Model file for the job. Use its own axes, mm. Coordinates: 2 decimals unless noted, no trailing zeros. Loops run counter-clockwise (first coordinate to the right, second up) from the corner with the lowest first, then second, coordinate; pieces in that order, holes last. Notation, with made-up numbers: (13, -24) -> (51, -24) arc R33 ccw to (51, 4) -> close; hole circle Ø3 at (30.5, 41). An arc over 180 degrees is marked (long way). Use one line per item in the form item = value.
```python
from build123d import *

# Parameters (mm, degrees)
BOSS_EXTRUDE1_DEPTH     = 25.4
F_1_4_CLEARANCE_HOLE1_D = 6.7564


with BuildPart() as part:
    # Sketch1 → Boss-Extrude1 (new body)
    with BuildSketch(Plane(origin=(0, 0, 0), x_dir=(1, 0, 0), z_dir=(0, 1, 0))):
        with BuildLine():
            Line((-63.5, -66.675), (63.5, -66.675))
            ThreePointArc((63.5, -66.675), (67.990128061, -64.815128061), (69.85, -60.325))
            Line((69.85, -60.325), (69.85, 60.325))
            ThreePointArc((69.85, 60.325), (67.990128061, 64.815128061), (63.5, 66.675))
            Line((63.5, 66.675), (-63.5, 66.675))
            ThreePointArc((-63.5, 66.675), (-67.990128061, 64.815128061), (-69.85, 60.325))
            Line((-69.85, 60.325), (-69.85, -60.325))
            ThreePointArc((-69.85, -60.325), (-67.990128061, -64.815128061), (-63.5, -66.675))
        make_face()
        with BuildLine():
            Line((-55.5625, 41.275), (-33.3375, 41.275))
            ThreePointArc((-33.3375, 41.275), (-32.214967985, 41.739967985), (-31.75, 42.8625))
            Line((-31.75, 42.8625), (-31.75, 52.3875))
            ThreePointArc((-31.75, 52.3875), (-32.214967985, 53.510032015), (-33.3375, 53.975))
            Line((-33.3375, 53.975), (-55.5625, 53.975))
            ThreePointArc((-55.5625, 53.975), (-56.685032015, 53.510032015), (-57.15, 52.3875))
            Line((-57.15, 52.3875), (-57.15, 42.8625))
            ThreePointArc((-57.15, 42.8625), (-56.685032015, 41.739967985), (-55.5625, 41.275))
        make_face(mode=Mode.SUBTRACT)
        with BuildLine():
            Line((-12.7, 42.8625), (-12.7, 52.3875))
            ThreePointArc((-12.7, 52.3875), (-12.235032015, 53.510032015), (-11.1125, 53.975))
            Line((-11.1125, 53.975), (11.1125, 53.975))
            ThreePointArc((11.1125, 53.975), (12.235032015, 53.510032015), (12.7, 52.3875))
            Line((12.7, 52.3875), (12.7, 42.8625))
            ThreePointArc((12.7, 42.8625), (12.235032015, 41.739967985), (11.1125, 41.275))
            Line((11.1125, 41.275), (-11.1125, 41.275))
            ThreePointArc((-11.1125, 41.275), (-12.235032015, 41.739967985), (-12.7, 42.8625))
        make_face(mode=Mode.SUBTRACT)
        with BuildLine():
            Line((31.75, 42.8625), (31.75, 52.3875))
            ThreePointArc((31.75, 52.3875), (32.214967985, 53.510032015), (33.3375, 53.975))
            Line((33.3375, 53.975), (55.5625, 53.975))
            ThreePointArc((55.5625, 53.975), (56.685032015, 53.510032015), (57.15, 52.3875))
            Line((57.15, 52.3875), (57.15, 42.8625))
            ThreePointArc((57.15, 42.8625), (56.685032015, 41.739967985), (55.5625, 41.275))
            Line((55.5625, 41.275), (33.3375, 41.275))
            ThreePointArc((33.3375, 41.275), (32.214967985, 41.739967985), (31.75, 42.8625))
        make_face(mode=Mode.SUBTRACT)
        with BuildLine():
            Line((-57.15, 11.1125), (-57.15, 20.6375))
            ThreePointArc((-57.15, 20.6375), (-56.685032015, 21.760032015), (-55.5625, 22.225))
            Line((-55.5625, 22.225), (-33.3375, 22.225))
            ThreePointArc((-33.3375, 22.225), (-32.214967985, 21.760032015), (-31.75, 20.6375))
            Line((-31.75, 20.6375), (-31.75, 11.1125))
            ThreePointArc((-31.75, 11.1125), (-32.214967985, 9.989967985), (-33.3375, 9.525))
            Line((-33.3375, 9.525), (-55.5625, 9.525))
            ThreePointArc((-55.5625, 9.525), (-56.685032015, 9.989967985), (-57.15, 11.1125))
        make_face(mode=Mode.SUBTRACT)
        with BuildLine():
            Line((-12.7, 11.1125), (-12.7, 20.6375))
            ThreePointArc((-12.7, 20.6375), (-12.235032015, 21.760032015), (-11.1125, 22.225))
            Line((-11.1125, 22.225), (11.1125, 22.225))
            ThreePointArc((11.1125, 22.225), (12.235032015, 21.760032015), (12.7, 20.6375))
            Line((12.7, 20.6375), (12.7, 11.1125))
            ThreePointArc((12.7, 11.1125), (12.235032015, 9.989967985), (11.1125, 9.525))
            Line((11.1125, 9.525), (-11.1125, 9.525))
            ThreePointArc((-11.1125, 9.525), (-12.235032015, 9.989967985), (-12.7, 11.1125))
        make_face(mode=Mode.SUBTRACT)
        with BuildLine():
            Line((31.75, 11.1125), (31.75, 20.6375))
            ThreePointArc((31.75, 20.6375), (32.214967985, 21.760032015), (33.3375, 22.225))
            Line((33.3375, 22.225), (55.5625, 22.225))
            ThreePointArc((55.5625, 22.225), (56.685032015, 21.760032015), (57.15, 20.6375))
            Line((57.15, 20.6375), (57.15, 11.1125))
            ThreePointArc((57.15, 11.1125), (56.685032015, 9.989967985), (55.5625, 9.525))
            Line((55.5625, 9.525), (33.3375, 9.525))
            ThreePointArc((33.3375, 9.525), (32.214967985, 9.989967985), (31.75, 11.1125))
        make_face(mode=Mode.SUBTRACT)
        with BuildLine():
            Line((-57.15, -20.6375), (-57.15, -11.1125))
            ThreePointArc((-57.15, -11.1125), (-56.685032015, -9.989967985), (-55.5625, -9.525))
            Line((-55.5625, -9.525), (-33.3375, -9.525))
            ThreePointArc((-33.3375, -9.525), (-32.214967985, -9.989967985), (-31.75, -11.1125))
            Line((-31.75, -11.1125), (-31.75, -20.6375))
            ThreePointArc((-31.75, -20.6375), (-32.214967985, -21.760032015), (-33.3375, -22.225))
            Line((-33.3375, -22.225), (-55.5625, -22.225))
            ThreePointArc((-55.5625, -22.225), (-56.685032015, -21.760032015), (-57.15, -20.6375))
        make_face(mode=Mode.SUBTRACT)
        with BuildLine():
            Line((-12.7, -20.6375), (-12.7, -11.1125))
            ThreePointArc((-12.7, -11.1125), (-12.235032015, -9.989967985), (-11.1125, -9.525))
            Line((-11.1125, -9.525), (11.1125, -9.525))
            ThreePointArc((11.1125, -9.525), (12.235032015, -9.989967985), (12.7, -11.1125))
            Line((12.7, -11.1125), (12.7, -20.6375))
            ThreePointArc((12.7, -20.6375), (12.235032015, -21.760032015), (11.1125, -22.225))
            Line((11.1125, -22.225), (-11.1125, -22.225))
            ThreePointArc((-11.1125, -22.225), (-12.235032015, -21.760032015), (-12.7, -20.6375))
        make_face(mode=Mode.SUBTRACT)
        with BuildLine():
            Line((31.75, -20.6375), (31.75, -11.1125))
            ThreePointArc((31.75, -11.1125), (32.214967985, -9.989967985), (33.3375, -9.525))
            Line((33.3375, -9.525), (55.5625, -9.525))
            ThreePointArc((55.5625, -9.525), (56.685032015, -9.989967985), (57.15, -11.1125))
            Line((57.15, -11.1125), (57.15, -20.6375))
            ThreePointArc((57.15, -20.6375), (56.685032015, -21.760032015), (55.5625, -22.225))
            Line((55.5625, -22.225), (33.3375, -22.225))
            ThreePointArc((33.3375, -22.225), (32.214967985, -21.760032015), (31.75, -20.6375))
        make_face(mode=Mode.SUBTRACT)
        with BuildLine():
            Line((-57.15, -52.3875), (-57.15, -42.8625))
            ThreePointArc((-57.15, -42.8625), (-56.685032015, -41.739967985), (-55.5625, -41.275))
            Line((-55.5625, -41.275), (-33.3375, -41.275))
            ThreePointArc((-33.3375, -41.275), (-32.214967985, -41.739967985), (-31.75, -42.8625))
            Line((-31.75, -42.8625), (-31.75, -52.3875))
            ThreePointArc((-31.75, -52.3875), (-32.214967985, -53.510032015), (-33.3375, -53.975))
            Line((-33.3375, -53.975), (-55.5625, -53.975))
            ThreePointArc((-55.5625, -53.975), (-56.685032015, -53.510032015), (-57.15, -52.3875))
        make_face(mode=Mode.SUBTRACT)
        with BuildLine():
            Line((-12.7, -52.3875), (-12.7, -42.8625))
            ThreePointArc((-12.7, -42.8625), (-12.235032015, -41.739967985), (-11.1125, -41.275))
            Line((-11.1125, -41.275), (11.1125, -41.275))
            ThreePointArc((11.1125, -41.275), (12.235032015, -41.739967985), (12.7, -42.8625))
            Line((12.7, -42.8625), (12.7, -52.3875))
            ThreePointArc((12.7, -52.3875), (12.235032015, -53.510032015), (11.1125, -53.975))
            Line((11.1125, -53.975), (-11.1125, -53.975))
            ThreePointArc((-11.1125, -53.975), (-12.235032015, -53.510032015), (-12.7, -52.3875))
        make_face(mode=Mode.SUBTRACT)
        with BuildLine():
            Line((31.75, -52.3875), (31.75, -42.8625))
            ThreePointArc((31.75, -42.8625), (32.214967985, -41.739967985), (33.3375, -41.275))
            Line((33.3375, -41.275), (55.5625, -41.275))
            ThreePointArc((55.5625, -41.275), (56.685032015, -41.739967985), (57.15, -42.8625))
            Line((57.15, -42.8625), (57.15, -52.3875))
            ThreePointArc((57.15, -52.3875), (56.685032015, -53.510032015), (55.5625, -53.975))
            Line((55.5625, -53.975), (33.3375, -53.975))
            ThreePointArc((33.3375, -53.975), (32.214967985, -53.510032015), (31.75, -52.3875))
        make_face(mode=Mode.SUBTRACT)
    extrude(amount=BOSS_EXTRUDE1_DEPTH)

    # 1/4 Clearance Hole1 (through all)
    with Locations(Plane(origin=(-63.5, 25.4, -60.325), x_dir=(0, 0, 1), z_dir=(0, 1, 0))):
        with Locations((0, 0), (0, 127), (120.65, 127), (120.65, 0), (60.325, 63.5), (0, 63.5), (120.65, 63.5)):
            Hole(F_1_4_CLEARANCE_HOLE1_D / 2)


solid = part.part
```
Q1. Wall check: line 1 along Z through (x, y) = (51, 4.5) (3 decimals); line 2 along X through (y, z) = (13.75, 51); line 3 along Z through (x, y) = (-33, 20.25) (3 decimals). Give the ranges that are in metal, low to high.
Result:
line_1 = -66.675 to -53.975, -41.275 to -22.225, -9.525 to 9.525, 22.225 to 41.275, 53.975 to 66.675
line_2 = -69.85 to -57.15, -31.75 to -12.7, 12.7 to 31.75, 57.15 to 69.85
line_3 = -66.675 to -53.939, -41.311 to -22.189, -9.561 to 9.561, 22.189 to 41.311, 53.939 to 66.675
Q2. Mould opens along Z. For faces 1 (the face through (0.1, 12.5, 63.7)), 2 (the face through (-68.039, 12.522, 64.765)), 3 (the face through (68.039, 12.522, -64.765)) say: released by +Z, released by -Z, zero draft, split by the parting line, or undercut.
Result:
face_1 = undercut
face_2 = released by +Z
face_3 = released by -Z
Q3. Band-saw the part on C-C, the plane z = 0. Write the cut outline in (x, y).
Result:
outline = (-69.85, 0) -> (-3.38, 0) -> (-3.38, 25.4) -> (-69.85, 25.4) -> close; (3.38, 0) -> (69.85, 0) -> (69.85, 25.4) -> (3.38, 25.4) -> close
Q4. Band-saw the part on D-D, the plane y = 19.75. State how many separate pieces and enclosed holes the cut face has, and give its area (3 significant figures).
Result:
separate_pieces = 1
enclosed_holes = 19
area = 14,500 mm2
Q5. Band-saw the part on B-B, the plane z = 14.5. Write the cut outline in (x, y), and give its area (3 significant figures).
Result:
outline = (-69.85, 0) -> (-57.15, 0) -> (-57.15, 25.4) -> (-69.85, 25.4) -> close; (-31.75, 0) -> (-12.7, 0) -> (-12.7, 25.4) -> (-31.75, 25.4) -> close; (12.7, 0) -> (31.75, 0) -> (31.75, 25.4) -> (12.7, 25.4) -> close; (57.15, 0) -> (69.85, 0) -> (69.85, 25.4) -> (57.15, 25.4) -> close
area = 1,610 mm2
Q6. Band-saw the part on A-A, the plane x = -6.5. Write the cut outline in (y, z) (3 decimals).
Result:
outline = (0, -66.675) -> (25.4, -66.675) -> (25.4, -53.975) -> (0, -53.975) -> close; (0, -41.275) -> (25.4, -41.275) -> (25.4, -22.225) -> (0, -22.225) -> close; (0, -9.525) -> (25.4, -9.525) -> (25.4, 9.525) -> (0, 9.525) -> close; (0, 22.225) -> (25.4, 22.225) -> (25.4, 41.275) -> (0, 41.275) -> close; (0, 53.975) -> (25.4, 53.975) -> (25.4, 66.675) -> (0, 66.675) -> close
